Here's the drawing with two shaded views (mm, measured from the low corner). I have some questions. Coordinates: 2 decimals unless noted, no trailing zeros. Write each loop counter-clockwise with the first axis right and the second up, starting at its lowest first coordinate (ties: lowest second). Pieces come first, ordered by that corner, then holes. Notation, with made-up numbers: M -36,12 L -11,12 A32 ccw -11,40 Z; hole C 72.5,28 d11. An arc over 180 degrees is marked long. Answer as CSV lines item,"result". Start each with the question number.
Item 1: Suppose I cut it at B-B, the plane z = 56. Write out the boundary of the cut face in (x, y) (3 decimals).
Item 2: If I drill on line 1 along Z through (x, y) = (4, 0.85) (3 decimals); line 2 along X through (y, z) = (1.2, 2) (3 decimals); line 3 along X through (y, z) = (2.6, 55.5), over which ranges is the centre line in solid material (lowest first)? Write a range as [from, to].
Item 3: Suppose I cut it at A-A, the plane x = 76. Write out the boundary of the cut face in (y, z) (3 decimals), and give its area (3 significant figures).
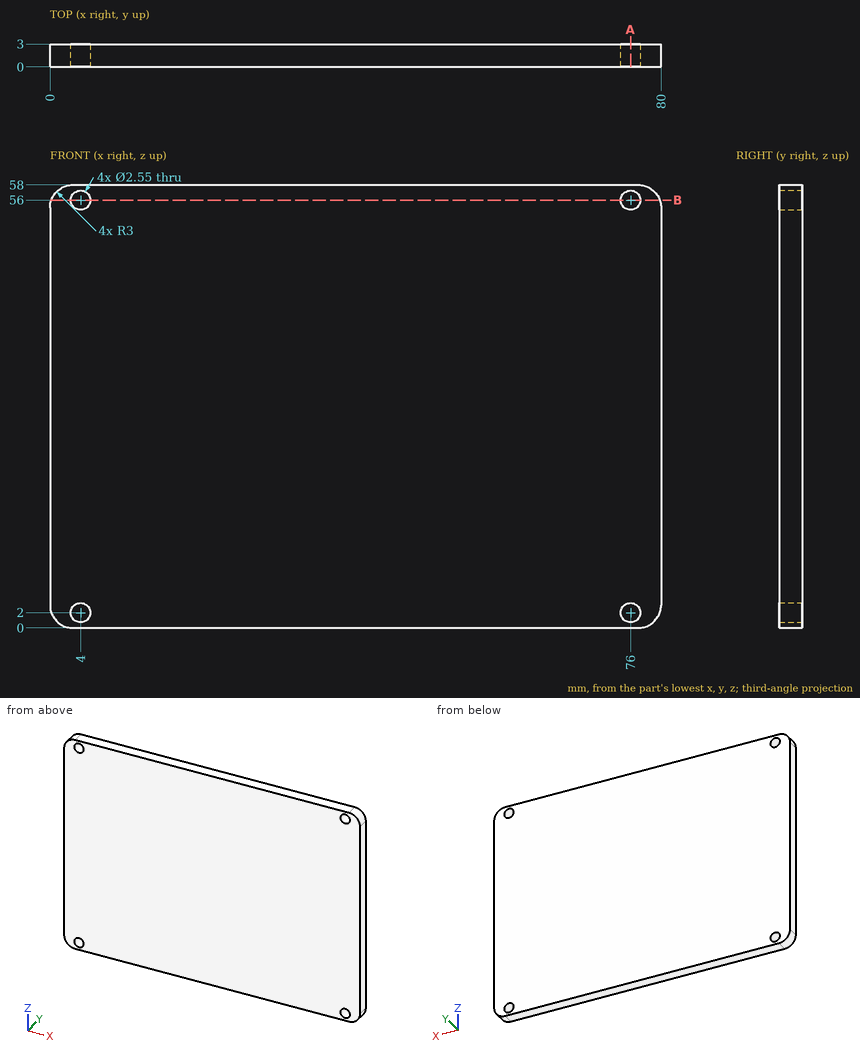
Ans:
1,outline,"M 0.172,0 L 2.725,0 L 2.725,3 L 0.172,3 Z; M 5.275,0 L 74.725,0 L 74.725,3 L 5.275,3 Z; M 77.275,0 L 79.828,0 L 79.828,3 L 77.275,3 Z"
2,line 1,"z = [0, 0.725], [3.275, 54.725], [57.275, 58]"
2,line 2,"x = [0.172, 2.725], [5.275, 74.725], [77.275, 79.828]"
2,line 3,"x = [0.04, 2.83], [5.17, 74.83], [77.17, 79.96]"
3,outline,"M 0,0 L 3,0 L 3,0.725 L 0,0.725 Z; M 0,3.275 L 3,3.275 L 3,54.725 L 0,54.725 Z; M 0,57.275 L 3,57.275 L 3,58 L 0,58 Z"
3,area,"159 mm^2"
